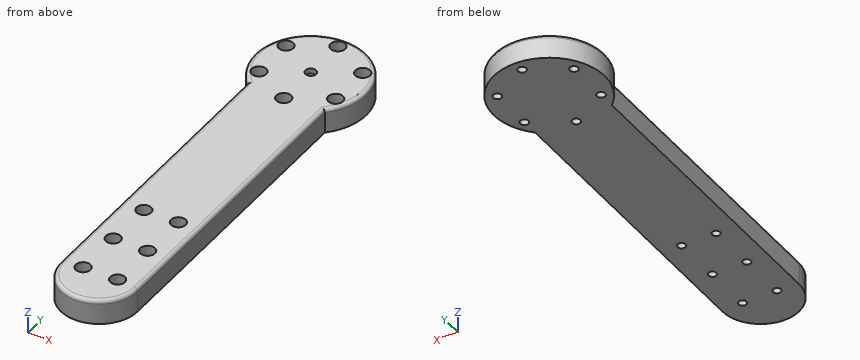
```python
from build123d import *

# Parameters (mm, degrees)
SKETCH_1_R          = 22.5
SKETCH_1_R_2        = 1.7
EXTRUDE_1_DEPTH     = 10
EXTRUDE_2_DEPTH     = 10
FILLET_1_R          = 1.5
SKETCH_3_R          = 1.6
CUT_EXTRUDE_1_DEPTH = 159.216092453
SKETCH_5_R          = 2.2
CUT_EXTRUDE_2_DEPTH = 2.2
SKETCH_6_R          = 3
CUT_EXTRUDE_3_DEPTH = 5


# Read off the part's stored shape, not the designer's step: 凸台-拉伸2
with BuildPart() as part:
    # 草图1 → 凸台-拉伸1 (new body)
    with BuildSketch(Plane.XY):
        Circle(SKETCH_1_R)
        with Locations((-15.588457268, 9)):
            Circle(SKETCH_1_R_2, mode=Mode.SUBTRACT)
        with Locations((0, 18)):
            Circle(SKETCH_1_R_2, mode=Mode.SUBTRACT)
        with Locations((15.588457268, 9)):
            Circle(SKETCH_1_R_2, mode=Mode.SUBTRACT)
        with Locations((15.588457268, -9)):
            Circle(SKETCH_1_R_2, mode=Mode.SUBTRACT)
        with Locations((0, -18)):
            Circle(SKETCH_1_R_2, mode=Mode.SUBTRACT)
        with Locations((-15.588457268, -9)):
            Circle(SKETCH_1_R_2, mode=Mode.SUBTRACT)
    extrude(amount=EXTRUDE_1_DEPTH)

    # 凸台-拉伸2 outline → 凸台-拉伸2 (add)
    with BuildSketch(Plane.XY):
        with BuildLine():
            Line((15.588457268, -140.7), (15.588457268, -16.22498074))
            ThreePointArc((15.588457268, -16.22498074), (0, -22.5), (-15.588457268, -16.22498074))
            Line((-15.588457268, -16.22498074), (-15.588457268, -140.7))
            ThreePointArc((-15.588457268, -140.7), (0, -156.288457268), (15.588457268, -140.7))
        make_face()
    extrude(amount=EXTRUDE_2_DEPTH)

    # 圆角1
    fillet_1_edges = [part.edges().sort_by_distance(p)[0] for p in [
        (0, 22.5, 10),
        (15.588457268, -78.46249037, 10),
        (-15.588457268, -78.46249037, 10),
        (0, -156.288457268, 10),
    ]]
    fillet(fillet_1_edges, radius=FILLET_1_R)

    # 草图3 → 切除-拉伸1 (cut, through all)
    with BuildSketch(Plane.XY.offset(10)):
        with Locations((7.266515313, -100.001775839)):
            Circle(SKETCH_3_R)
        with Locations((-6.733484478, -100)):
            Circle(SKETCH_3_R)
        with Locations((7, -120)):
            Circle(SKETCH_3_R)
        with Locations((7, -140)):
            Circle(SKETCH_3_R)
        with Locations((-7, -140)):
            Circle(SKETCH_3_R)
        with Locations((-7, -120)):
            Circle(SKETCH_3_R)
    extrude(amount=-CUT_EXTRUDE_1_DEPTH, mode=Mode.SUBTRACT)

    # 草图5 → 切除-拉伸2 (cut)
    with BuildSketch(Plane.XY.offset(10)):
        Circle(SKETCH_5_R)
    extrude(amount=-CUT_EXTRUDE_2_DEPTH, mode=Mode.SUBTRACT)

    # 草图6 → 切除-拉伸3 (cut)
    with BuildSketch(Plane.XY.offset(10)):
        with Locations((-15.588457268, -9)):
            Circle(SKETCH_6_R)
        with Locations((0, -18)):
            Circle(SKETCH_6_R)
        with Locations((15.588457268, -9)):
            Circle(SKETCH_6_R)
        with Locations((15.588457268, 9)):
            Circle(SKETCH_6_R)
        with Locations((0, 18)):
            Circle(SKETCH_6_R)
        with Locations((-15.588457268, 9)):
            Circle(SKETCH_6_R)
        with Locations((-6.733484478, -100)):
            Circle(SKETCH_6_R)
        with Locations((7.266515313, -100.001775839)):
            Circle(SKETCH_6_R)
        with Locations((7, -120)):
            Circle(SKETCH_6_R)
        with Locations((-7, -120)):
            Circle(SKETCH_6_R)
        with Locations((-7, -140)):
            Circle(SKETCH_6_R)
        with Locations((7, -140)):
            Circle(SKETCH_6_R)
    extrude(amount=-CUT_EXTRUDE_3_DEPTH, mode=Mode.SUBTRACT)


solid = part.part
```
For this review, take the finished solid that the model builds, in its own axes (mm). Coordinates: 2 decimals unless noted, no trailing zeros. Write each loop counter-clockwise with the first axis right and the second up, starting at its lowest first coordinate (ties: lowest second). Pieces come first, ordered by that corner, then holes. Notation, with made-up numbers: (10, 85.5) -> (46, 85.5) arc R7 cw to (46, 97.5) -> close; hole circle Ø1 at (71, 25.5). An arc over 180 degrees is marked (long way). Put each result on its own line as item: value.
Q1. Take a section at A-A, the plane y = -120. State the section outline as (x, z) points.
From the geometry:
outline: (-15.59, 0) -> (-8.6, 0) -> (-8.6, 5) -> (-10, 5) -> (-10, 10) -> (-14.09, 10) arc R1.5 ccw to (-15.59, 8.5) -> close; (-5.4, 0) -> (5.4, 0) -> (5.4, 5) -> (4, 5) -> (4, 10) -> (-4, 10) -> (-4, 5) -> (-5.4, 5) -> close; (8.6, 0) -> (15.59, 0) -> (15.59, 8.5) arc R1.5 ccw to (14.09, 10) -> (10, 10) -> (10, 5) -> (8.6, 5) -> close
Q2. Wall thickness on L1, parallel to X at y = -140, z = 6.5; L2, parallel to Y at x = 0, z = 5.5; L3, parallel to X at y = -120, z = 1.05: over which ranges is each line inside the solid? List them lowest first.
From the geometry:
L1: x = -15.59 to -10, -4 to 4, 10 to 15.59
L2: y = -156.29 to -21, -15 to 15, 21 to 22.5
L3: x = -15.59 to -8.6, -5.4 to 5.4, 8.6 to 15.59
Q3. Clearance check with flat-ended pins moving along their axes: pin 1 Ø6 at (x, y) = (17, -104) entering from +Z; pin 2 Ø3 at (x, z) = (6.5, 2.5) entering from +Y; pin 3 Ø6 at (x, z) = (9.5, 3) entering from -Y; pin 4 Ø1 at (x, z) = (-12, 8) entering from +Y. State where each tip first meets the part, or that it passes through.
From the geometry:
pin 1: stops at z = 10
pin 2: stops at y = 21.94
pin 3: stops at y = -154.87
pin 4: stops at y = 19.34
Q4. Take a section at B-B, the plane z = 2. Count the separate pieces of the cut face and the enclosed holes in it, then the cut area to 3 significant figures.
From the geometry:
separate pieces: 1
enclosed holes: 12
area: 5,620 mm2
